For this review, take the finished solid that the model builds, in its own axes (mm). A direction names the side the tool comes from. Coordinates: 2 decimals unless noted, no trailing zeros. Loops run counter-clockwise (first coordinate to the right, second up) from the corner with the lowest first, then second, coordinate; pieces in that order, holes last. Notation, with made-up numbers: M 79.5,73.25 L 120.5,73.25 A20 ccw 120.5,82.25 Z; hole C 4,84 d1. An arc over 180 degrees is marked long. Use one line per item in the form item = value.
```python
from build123d import *

# Parameters (mm, degrees)
F0_W     = 5
F0_H     = 5
F1_DEPTH = 5
F7_W     = 175
F7_H     = 5
F7_W_2   = 5
F8_DEPTH = 0.9


with BuildPart() as f1:
    # F0 (on Top) → F1 (new body)
    with BuildSketch(Plane.XY):
        with Locations((2.5, 2.5)):
            Rectangle(F0_W, F0_H)
    extrude(amount=F1_DEPTH)



with BuildPart() as f2_1:
    # F2: copy of F1
    add(f1.part.moved(Location((15, 0, 0))))


with BuildPart() as f3_1:
    # F3: copy of F2_1
    add(f2_1.part.moved(Location((25, 0, 0))))


with BuildPart() as f4_1:
    # F4: copy of F3_1
    add(f3_1.part.moved(Location((35, 0, 0))))


with BuildPart() as f5_1:
    # F5: copy of F4_1
    add(f4_1.part.moved(Location((45, 0, 0))))


with BuildPart() as f6_1:
    # F6: copy of F5_1
    add(f5_1.part.moved(Location((55, 0, 0))))


with BuildPart() as f1_1:
    add(f1.part)

    add(f2_1.part)  # F8 merges F2_1

    add(f3_1.part)  # F8 merges F3_1

    add(f4_1.part)  # F8 merges F4_1

    add(f5_1.part)  # F8 merges F5_1

    add(f6_1.part)  # F8 merges F6_1
    # F7 (on face) → F8 (join)
    with BuildSketch(Plane.XY.offset(5)):
        with Locations((92.5, 2.5)):
            Rectangle(F7_W, F7_H)
        with Locations((2.5, 2.5)):
            Rectangle(F7_W_2, F7_H)
    extrude(amount=F8_DEPTH)


solid = f1_1.part
```
1. Draft analysis for pull direction X (two halves, no side actions). For faces 3 (the face through (2, 3, 0)), 4 (the face through (75, 2, 2)), 5 (the face through (120, 2, 2)), 6 (the face through (180, 2, 3)), state which applies: +X half, -X half, draft (parallel to the pull), parting line (faces both ways), or undercut.
Computed values:
face_3 = draft
face_4 = undercut
face_5 = undercut
face_6 = +X half
2. Consider section B-B on y = 1. Write out the cut boundary in (x, z).
Computed values:
outline = M 0,0 L 5,0 L 5,5 L 15,5 L 15,0 L 20,0 L 20,5 L 40,5 L 40,0 L 45,0 L 45,5 L 75,5 L 75,0 L 80,0 L 80,5 L 120,5 L 120,0 L 125,0 L 125,5 L 175,5 L 175,0 L 180,0 L 180,5.9 L 0,5.9 Z
3. Consider section C-C on x = 38. Write out the cut boundary in (y, z), plus the area to 3 significant figures.
Computed values:
outline = M 0,5 L 5,5 L 5,5.9 L 0,5.9 Z
area = 4.50 mm2
4. For pin 1 Ø1.5 at (x, y) = (103, 3) entering from -Z, flat-tipped, find the tip position at first contact; note if it passes through.
Computed values:
pin_1 = 5
5. Tool access review of faces 1 (the face through (20, 2, 2)), 2 (the face through (42, 3, 0)): name each direction out of +Z, -Z, +X, -X, +Y, -Y from which nothing blocks a thin tool from reaching the whole face with its end or side.
Computed values:
face_1 = -Z, +Y, -Y
face_2 = -Z, +X, -X, +Y, -Y
6. Wall thickness on line 1 along X through (y, z) = (2.5, 3.85); line 2 along Z through (x, y) = (130, 1.8): over which ranges is each line inside the solid? List them lowest first. Write a range as from..to.
Computed values:
line_1 = 0..5, 15..20, 40..45, 75..80, 120..125, 175..180
line_2 = 5..5.9
7. Consider section A-A on z = 1.15. Write out the cut boundary in (x, y), plus the area to 3 significant figures.
Computed values:
outline = M 0,0 L 5,0 L 5,5 L 0,5 Z; M 15,0 L 20,0 L 20,5 L 15,5 Z; M 40,0 L 45,0 L 45,5 L 40,5 Z; M 75,0 L 80,0 L 80,5 L 75,5 Z; M 120,0 L 125,0 L 125,5 L 120,5 Z; M 175,0 L 180,0 L 180,5 L 175,5 Z
area = 150 mm2
